from build123d import *

# Parameters (mm, degrees)
BOSS_EXTRUDE1_DEPTH = 3.175
BOSS_EXTRUDE2_DEPTH = 3.175
FILLET1_R           = 6.35
SKETCH3_R           = 2.286
CUT_EXTRUDE1_DEPTH  = 518.046822543
FILLET2_R           = 1.5875
SCALE4_SCALE        = 0.9


with BuildPart() as part:
    # Sketch1 → Boss-Extrude1 (new body)
    with BuildSketch(Plane.XY):
        with BuildLine():
            Line((192.983759728, 175.441215803), (96.309561297, 130.227436844))
            ThreePointArc((96.309561297, 130.227436844), (87.484677999, 126.692854878), (78.317465574, 124.176100766))
            ThreePointArc((78.317465574, 124.176100766), (74.466708454, 122.444126875), (71.664680309, 119.285535064))
            ThreePointArc((71.664680309, 119.285535064), (70.058699462, 115.330377605), (69.512486748, 111.096691661))
            ThreePointArc((69.512486748, 111.096691661), (72.264254662, 99.39829615), (79.935173725, 90.147259184))
            ThreePointArc((79.935173725, 90.147259184), (88.679137799, 87.2113543), (97.423101873, 90.147259184))
            ThreePointArc((97.423101873, 90.147259184), (105.809954176, 95.76246485), (114.789367372, 100.371148488))
            Line((114.789367372, 100.371148488), (237.663968602, 154.698817321))
            Line((237.663968602, 154.698817321), (360.538569833, 100.371148488))
            ThreePointArc((360.538569833, 100.371148488), (369.517983029, 95.76246485), (377.904835332, 90.147259184))
            ThreePointArc((377.904835332, 90.147259184), (386.648799405, 87.2113543), (395.392763479, 90.147259184))
            ThreePointArc((395.392763479, 90.147259184), (403.063682542, 99.39829615), (405.815450457, 111.096691661))
            ThreePointArc((405.815450457, 111.096691661), (405.269237742, 115.330377605), (403.663256896, 119.285535064))
            ThreePointArc((403.663256896, 119.285535064), (400.86122875, 122.444126875), (397.01047163, 124.176100766))
            ThreePointArc((397.01047163, 124.176100766), (387.843259205, 126.692854878), (379.018375907, 130.227436844))
            Line((379.018375907, 130.227436844), (282.344177476, 175.441215803))
            Line((282.344177476, 175.441215803), (318.55970852, 192.243538611))
            ThreePointArc((318.55970852, 192.243538611), (327.615304884, 192.094216272), (336.396188974, 194.312818822))
            Line((336.396188974, 194.312818822), (352.546314681, 200.753440043))
            ThreePointArc((352.546314681, 200.753440043), (399.763650832, 176.34843342), (441.305300897, 143.191646915))
            ThreePointArc((441.305300897, 143.191646915), (423.803151272, 189.77617727), (389.079447428, 225.423170147))
            ThreePointArc((389.079447428, 225.423170147), (386.452648862, 232.479391977), (381.864833782, 238.449508393))
            ThreePointArc((381.864833782, 238.449508393), (373.00378877, 245.841981415), (363.187253088, 251.908479853))
            ThreePointArc((363.187253088, 251.908479853), (353.665803765, 254.648371797), (343.834991341, 253.415435392))
            ThreePointArc((343.834991341, 253.415435392), (292.266671735, 267.690958579), (238.759580195, 267.420211094))
            ThreePointArc((238.759580195, 267.420211094), (274.672718132, 253.0886387), (307.794144835, 233.135730718))
            ThreePointArc((307.794144835, 233.135730718), (301.585446406, 230.415438718), (297.431026809, 225.059253268))
            Line((297.431026809, 225.059253268), (237.663968602, 196.776891326))
            Line((237.663968602, 196.776891326), (177.896910395, 225.059253268))
            ThreePointArc((177.896910395, 225.059253268), (173.742490798, 230.415438718), (167.533792369, 233.135730718))
            ThreePointArc((167.533792369, 233.135730718), (200.655219072, 253.0886387), (236.568357009, 267.420211094))
            ThreePointArc((236.568357009, 267.420211094), (183.061265469, 267.690958579), (131.492945863, 253.415435392))
            ThreePointArc((131.492945863, 253.415435392), (121.66213344, 254.648371797), (112.140684116, 251.908479853))
            ThreePointArc((112.140684116, 251.908479853), (102.324148434, 245.841981415), (93.463103422, 238.449508393))
            ThreePointArc((93.463103422, 238.449508393), (88.875288342, 232.479391977), (86.248489776, 225.423170147))
            ThreePointArc((86.248489776, 225.423170147), (51.524785932, 189.77617727), (34.022636308, 143.191646915))
            ThreePointArc((34.022636308, 143.191646915), (75.564286372, 176.34843342), (122.781622523, 200.753440043))
            Line((122.781622523, 200.753440043), (138.931748231, 194.312818822))
            ThreePointArc((138.931748231, 194.312818822), (147.712632321, 192.094216272), (156.768228685, 192.243538611))
            Line((156.768228685, 192.243538611), (192.983759728, 175.441215803))
        make_face()
    extrude(amount=BOSS_EXTRUDE1_DEPTH)

    # Sketch2 → Boss-Extrude2 (add)
    with BuildSketch(Plane.XY):
        Polygon((124.775079826, 104.786222668), (124.775079826, 67.83365331), (350.552857378, 67.83365331), (350.552857378, 104.786222668), (304.455055516, 125.167864508), (288.463968602, 89.00031913), (186.863968602, 89.00031913), (170.872881688, 125.167864508), align=None)
    extrude(amount=BOSS_EXTRUDE2_DEPTH)

    # Fillet1
    fillet1_edges = [part.edges().sort_by_distance(p)[0] for p in [
        (304.455055516, 125.167864508, 1.5875),
        (350.552857378, 104.786222668, 1.5875),
        (350.552857378, 67.83365331, 1.5875),
        (124.775079826, 67.83365331, 1.5875),
        (124.775079826, 104.786222668, 1.5875),
        (170.872881688, 125.167864508, 1.5875),
    ]]
    fillet(fillet1_edges, radius=FILLET1_R)

    # Sketch3 → Cut-Extrude1 (cut, through all)
    with BuildSketch(Plane.XY.offset(3.175)):
        with Locations((237.663968602, 175.737854324)):
            Circle(SKETCH3_R)
        with Locations((78.913968602, 197.962854324)):
            Circle(SKETCH3_R)
        with Locations((174.163968602, 255.112854324)):
            Circle(SKETCH3_R)
        with Locations((301.163968602, 255.112854324)):
            Circle(SKETCH3_R)
        with Locations((396.413968602, 197.962854324)):
            Circle(SKETCH3_R)
        with Locations((148.763968602, 131.287854324)):
            Circle(SKETCH3_R)
        with Locations((326.563968602, 131.287854324)):
            Circle(SKETCH3_R)
    extrude(amount=-CUT_EXTRUDE1_DEPTH, mode=Mode.SUBTRACT)

    # Fillet2
    fillet2_edges = [part.edges().sort_by_distance(p)[0] for p in [
        (34.022636308, 143.191646915, 1.5875),
        (236.568357009, 267.420211094, 1.5875),
        (238.759580195, 267.420211094, 1.5875),
        (441.305300897, 143.191646915, 1.5875),
    ]]
    fillet(fillet2_edges, radius=FILLET2_R)


with BuildPart() as part_1:
    # Scale4: scaled about (237.663968386, 165.877309559, 1.5875)
    add(part.part.scale(SCALE4_SCALE).moved(Location((23.766396839, 16.587730956, 0.15875))))


solid = part_1.part
Verification items for the finished model (mm, model axes). A direction names the side the tool comes from. Coordinates: 2 decimals unless noted, no trailing zeros. Loops run counter-clockwise (first coordinate to the right, second up) from the corner with the lowest first, then second, coordinate; pieces in that order, holes last. Notation, with made-up numbers: M 76,83 L 107,83 A31 ccw 107,121 Z; hole C 53.25,-36 d11. An arc over 180 degrees is marked long. One line per item, written item: value.
1. Material ranges on line 1 along Y through (x, z) = (217.5, 1.85); line 2 along Y through (x, z) = (294.5, 1); line 3 along X through (y, z) = (152.5, 0.95), recorded low to high. Write a range as from..to.
Answers follow:
line 1: 77.64..96.69, 146.9..203.23, 250.35..258.95
line 2: 77.64..121.83, 130.13..166.71, 182.2..223.38, 230.76..244.16, 248.22..256.31
line 3: 55.71..61.93, 150.44..230.16, 245.17..324.88, 413.4..419.62
2. Set-up check for faces 1 (the flat face through (235, 170, 0.159)), 2 (the cylindrical face through (356.22, 102.84, 1.57)), 3 (the flat face through (289.51, 110.54, 1.57)): record each of +Z, -Z, +X, -X, +Y, -Y from which the full face is reachable in a straight line by a thin tool's end or side.
Answers follow:
face 1: -Z, +X, -X, +Y, -Y
face 2: +Z, -Z, -Y
face 3: +Z, -Z
3. Section check D-D on y = 89.5. Record the cut outline in (x, z).
Answers follow:
outline: M 136.06,0.16 L 339.26,0.16 L 339.26,3.02 L 136.06,3.02 Z
4. Section check B-B on x = 265.5. Record the cut outline in (y, z), plus the area to 3 significant figures.
Answers follow:
outline: M 77.64,0.16 L 96.69,0.16 L 96.69,3.02 L 77.64,3.02 Z; M 143.51,0.16 L 206.86,0.16 L 206.86,3.02 L 143.51,3.02 Z; M 246.99,0.16 L 259.04,0.16 L 259.04,3.02 L 246.99,3.02 Z
area: 270 mm^2
5. Mould release check, pull along Y, two halves, no side actions. Record for faces 4 (the flat face through (235, 170, 3.016)), 5 (the cylindrical face through (295.262, 224.014, 1.567)), 6 (the cylindrical face through (103.8, 225.9, 1.6)): pulls with the +Y half, pulls with the -Y half, needs draft (parallel to the pull), parting line crosses it, or undercut.
Answers follow:
face 4: needs draft
face 5: undercut
face 6: pulls with the +Y half
6. Gauge pin test, flat ends, axial feed: P1, Ø4.5, axis at x = 317.67, y = 134.75, coming from the +Z side; P2, Ø3.5, axis at x = 94.79, y = 194.75, coming from the +Z side. Record the tip position at first contact, or that the pin passes through.
Answers follow:
P1: z = 3.02
P2: through
7. Section check A-A on y = 140.5. Record the cut outline in (x, z).
Answers follow:
outline: M 124.79,0.16 L 203.02,0.16 L 203.02,3.02 L 124.79,3.02 Z; M 272.31,0.16 L 350.54,0.16 L 350.54,3.02 L 272.31,3.02 Z
8. Section check C-C on x = 304.5. Record the cut outline in (y, z).
Answers follow:
outline: M 77.64,0.16 L 162.03,0.16 L 162.03,3.02 L 77.64,3.02 Z; M 186.84,0.16 L 254.22,0.16 L 254.22,3.02 L 186.84,3.02 Z
